Could you check a few things on this model? Use its own coordinates, in mm. A direction names the side the tool comes from. Round coordinates to 2 decimals unless told otherwise and drop trailing zeros. Loops run counter-clockwise (first coordinate to the right, second up) from the corner with the lowest first, then second, coordinate; pieces in that order, holes last. Notation, with made-up numbers: M -13,87 L 6,87 A28 cw 6,106 Z; hole C 53,20 d4. An arc over 180 degrees is marked long. Answer in a Markdown table with one row per item.
```python
from build123d import *

# Parameters (mm, degrees)
SKETCH1_W           = 125
SKETCH1_H           = 460
BOSS_EXTRUDE1_DEPTH = 33
SKETCH2_W           = 50
SKETCH2_H           = 15
CUT_EXTRUDE1_DEPTH  = 400


with BuildPart() as part:
    # Sketch1 → Boss-Extrude1 (new body)
    with BuildSketch(Plane.XY):
        with Locations((-62.5, -230)):
            Rectangle(SKETCH1_W, SKETCH1_H)
    extrude(amount=BOSS_EXTRUDE1_DEPTH)

    # Sketch2 → Cut-Extrude1 (cut)
    with BuildSketch(Plane(origin=(0, 0, 0), x_dir=(1, 0, 0), z_dir=(0, 1, 0))):
        with Locations((-25, -16.5)):
            Rectangle(SKETCH2_W, SKETCH2_H)
    extrude(amount=-CUT_EXTRUDE1_DEPTH, mode=Mode.SUBTRACT)


solid = part.part
```
1) If we mould it in two halves opening along Z, with no side actions, what happens to faces 3 (the face through (-25, -197, 9)), 4 (the face through (-63, -227, 0)), 5 (the face through (-125, -233, 16))? For each: released by +Z, released by -Z, zero draft, split by the parting line, or undercut.
Computed:
| item | result |
|---|---|
| face 3 | undercut |
| face 4 | released by -Z |
| face 5 | zero draft |
2) I need wall thicknesses on line 1 (Z direction, x = -38.5, y = -260.5); line 2 (X direction, y = -51, z = 11); line 3 (Y direction, x = -27, z = 15). Which ranges of each line are inside material? Lowest first, please.
Computed:
| item | result |
|---|---|
| line 1 | z = 0 to 9, 24 to 33 |
| line 2 | x = -125 to -50 |
| line 3 | y = -460 to -400 |
3) I want a section at A-A, the plane y = -223. Please give me the cut outline in (x, z).
Computed:
| item | result |
|---|---|
| outline | M -125,0 L 0,0 L 0,9 L -50,9 L -50,24 L 0,24 L 0,33 L -125,33 Z |
4) Will these pins go through, and if not, where does the flat tip stop? P1, Ø7.5, axis at x = -22, z = 17.5, coming from the +Y side; P2, Ø2, axis at y = -253.5, z = 29, coming from the +X side.
Computed:
| item | result |
|---|---|
| P1 | stops at y = -400 |
| P2 | stops at x = 0 |
5) Which directions (+Z, -Z, +X, -X, +Y, -Y) give clear straight access to the entire face, cutting with the end or side of a thin tool? Please do faces 1 (the face through (-25, -197, 24)), 2 (the face through (-63, -227, 33)).
Computed:
| item | result |
|---|---|
| face 1 | +X, +Y |
| face 2 | +Z, +X, -X, +Y, -Y |
6) I want a section at C-C, the plane z = 18.5. Please give me the cut outline in (x, y).
Computed:
| item | result |
|---|---|
| outline | M -125,-460 L 0,-460 L 0,-400 L -50,-400 L -50,0 L -125,0 Z |
7) I want a section at B-B, the plane x = -19. Please give me the cut outline in (y, z).
Computed:
| item | result |
|---|---|
| outline | M -460,0 L 0,0 L 0,9 L -400,9 L -400,24 L 0,24 L 0,33 L -460,33 Z |
